Build history of the part. All positions in model axes, mm. A direction names the side the tool comes from. Give positions to 0.01 mm unless a question says otherwise; leave off trailing zeros. Loops run counter-clockwise (first coordinate to the right, second up) from the corner with the lowest first, then second, coordinate; pieces in that order, holes last. Notation, with made-up numbers: M 77.5,57.25 L 93.5,57.25 A7 ccw 93.5,68.25 Z; hole C 69.5,39.5 d9. An arc over 180 degrees is marked long. Put each result on its own line as item: value.
```python
from build123d import *

# Parameters (mm, degrees)
BOSS_EXTRUDE1_DEPTH = 6.35
CUT_EXTRUDE1_DEPTH  = 6.35


with BuildPart() as part:
    # Sketch1 → Boss-Extrude1 (new body)
    with BuildSketch(Plane.XY):
        Polygon((0, 101.6), (0, 76.2), (44.45, 0), (120.65, 0), (165.1, 76.2), (165.1, 101.6), align=None)
    extrude(amount=BOSS_EXTRUDE1_DEPTH)

    # Sketch2 → Cut-Extrude1 (cut)
    with BuildSketch(Plane.XY.offset(6.35)):
        Polygon((38.1, 76.2), (127, 76.2), (127, 50.8), (96.613225755, 51.156306651), (95.25, 50.8), (95.25, 0), (69.85, 0), (69.85, 50.8), (38.1, 50.8), align=None)
    extrude(amount=-CUT_EXTRUDE1_DEPTH, mode=Mode.SUBTRACT)


solid = part.part
```
Q1. Slice it at C-C (z = 4). List the corners of the cut face in (x, y), and give its area (3 significant figures).
Here are the results:
outline: M 0,76.2 L 44.45,0 L 69.85,0 L 69.85,50.8 L 38.1,50.8 L 38.1,76.2 L 127,76.2 L 127,50.8 L 96.61,51.16 L 95.25,50.8 L 95.25,0 L 120.65,0 L 165.1,76.2 L 165.1,101.6 L 0,101.6 Z
area: 9,840 mm²
Q2. Slice it at A-A (x = 56). List the corners of the cut face in (y, z).
Here are the results:
outline: M 0,0 L 50.8,0 L 50.8,6.35 L 0,6.35 Z; M 76.2,0 L 101.6,0 L 101.6,6.35 L 76.2,6.35 Z
Q3. Slice it at D-D (x = 74.5). List the corners of the cut face in (y, z).
Here are the results:
outline: M 76.2,0 L 101.6,0 L 101.6,6.35 L 76.2,6.35 Z
Q4. Slice it at B-B (y = 10). List the corners of the cut face in (x, z).
Here are the results:
outline: M 38.62,0 L 69.85,0 L 69.85,6.35 L 38.62,6.35 Z; M 95.25,0 L 126.48,0 L 126.48,6.35 L 95.25,6.35 Z
Q5. Drop flat-ended pins along their axis: pin 1 Ø1.9 at (x, z) = (78.5, 2) entering from -Y; pin 2 Ø3 at (y, z) = (70, 4) entering from +X; pin 3 Ø4 at (x, y) = (18, 57.5) entering from -Z; pin 4 Ø1 at (y, z) = (22, 3) entering from +X (3 decimals). Give the stop position or say it passes through.
Here are the results:
pin 1: y = 76.2
pin 2: x = 162.36
pin 3: z = 0
pin 4: x = 133.775
Q6. Probe line 1 (Y direction, x = 85, z = 0.5); line 2 (Y direction, x = 47.5, z = 2.25); line 3 (X direction, y = 42, z = 1.25). List the from-to ranges inside material, lowest first. Write a range as from..to.
Here are the results:
line 1: 76.2..101.6
line 2: 0..50.8, 76.2..101.6
line 3: 19.95..69.85, 95.25..145.15
Q7. Tool access for faces 4 (the flat face through (0, 89, 3)), 5 (the flat face through (38.1, 63, 3)), 6 (the flat face through (95.25, 26, 3)): list every direction of +Z, -Z, +X, -X, +Y, -Y with a clear straight run to the whole face (end or side of a thin tool).
Here are the results:
face 4: +Z, -Z, -X, +Y, -Y
face 5: +Z, -Z
face 6: +Z, -Z, -Y
Q8. Mould opens along Y. For faces 1 (the flat face through (127, 64, 3)), 2 (the flat face through (100, 40, 6.35)), 3 (the flat face through (142.564, 37.567, 3.131)) say: pulls with the +Y half, pulls with the -Y half, needs draft (parallel to the pull), parting line crosses it, or undercut.
Here are the results:
face 1: undercut
face 2: needs draft
face 3: pulls with the -Y half
